CAD build for the part. Positions are in the model's coordinates, mm. A direction names the side the tool comes from. Round coordinates to 2 decimals unless told otherwise and drop trailing zeros. Loops run counter-clockwise (first coordinate to the right, second up) from the corner with the lowest first, then second, coordinate; pieces in that order, holes last. Notation, with made-up numbers: (77.5, 49.25) -> (127.5, 49.25) arc R22 ccw to (127.5, 68.25) -> close; hole circle Ø3 at (25.5, 20.5). An arc over 180 degrees is marked (long way). Answer as CSV lines item,"result".
```python
from build123d import *

# Parameters (mm, degrees)
F0_R     = 2.75
F1_DEPTH = 7
F2_R     = 2.75
F2_R_2   = 2.5
F3_DEPTH = 6
F4_R     = 2.75
F4_R_2   = 2.5
F5_DEPTH = 6


with BuildPart() as f1:
    # F0 (on Front) → F1 (new body, symmetric)
    with BuildSketch(Plane.XZ):
        Circle(F0_R)
    extrude(amount=F1_DEPTH, both=True)

    # F2 (on face) → F3 (cut)
    with BuildSketch(Plane.XZ.offset(7)):
        Circle(F2_R)
        Circle(F2_R_2, mode=Mode.SUBTRACT)
    extrude(amount=-F3_DEPTH, mode=Mode.SUBTRACT)

    # F4 (on Front) → F5 (cut)
    with BuildSketch(Plane.XZ):
        Circle(F4_R)
        Circle(F4_R_2, mode=Mode.SUBTRACT)
    extrude(amount=-F5_DEPTH, mode=Mode.SUBTRACT)


solid = f1.part
```
Q1. Tool access for faces 1 (the cylindrical face through (-0.54, 2.96, -2.44)), 2 (the cylindrical face through (-0.54, -4.04, -2.44)), 3 (the cylindrical face through (-0.596, 6.493, -2.685)): list every direction of +Z, -Z, +X, -X, +Y, -Y with a clear straight run to the whole face (end or side of a thin tool).
Results:
face 1,"none"
face 2,"-Y"
face 3,"+Y, -Y"
Q2. Probe L1, parallel to Y at x = -1.6, z = 2; L2, parallel to X at y = -4, z = -0.1; L3, parallel to X at y = 3, z = -1.35. List the from-to ranges inside material, lowest first. Write a range as [from, to].
Results:
L1,"[-1, 0], [6, 7]"
L2,"[-2.5, 2.5]"
L3,"[-2.1, 2.1]"
Q3. Slice it at B-B, the plane z = 0. Give the cut face in (x, y).
Results:
outline,"(-2.75, -1) -> (-2.5, -1) -> (-2.5, -7) -> (2.5, -7) -> (2.5, -1) -> (2.75, -1) -> (2.75, 0) -> (2.5, 0) -> (2.5, 6) -> (2.75, 6) -> (2.75, 7) -> (-2.75, 7) -> (-2.75, 6) -> (-2.5, 6) -> (-2.5, 0) -> (-2.75, 0) -> close"
Q4. Drop flat-ended pins along their axis: pin 1 Ø1.5 at (x, y) = (-2, 4) entering from -Z; pin 2 Ø2 at (y, z) = (0, 1.5) entering from -X; pin 3 Ø1.5 at (x, y) = (2, 0.5) entering from -Z. Give the stop position or say it passes through.
Results:
pin 1,"z = -2.17"
pin 2,"x = -2.7"
pin 3,"z = -2.34"
Q5. Slice it at A-A, the plane x = 0. Give the cut face in (y, z).
Results:
outline,"(-7, -2.5) -> (-1, -2.5) -> (-1, -2.75) -> (0, -2.75) -> (0, -2.5) -> (6, -2.5) -> (6, -2.75) -> (7, -2.75) -> (7, 2.75) -> (6, 2.75) -> (6, 2.5) -> (0, 2.5) -> (0, 2.75) -> (-1, 2.75) -> (-1, 2.5) -> (-7, 2.5) -> close"
Q6. Slice it at C-C, the plane y = -2.5. Give the cut face in (x, z).
Results:
outline,"circle Ø5 at (0, 0)"
